Can you work these out from the model? Positions are in its coordinate system, mm. A direction names the side the tool comes from. Round coordinates to 2 decimals unless told otherwise and drop trailing zeros. Order: outer loops, then holes, each group sorted by start corner. A loop starts at its lowest first (then second) coordinate and runs counter-clockwise, first axis right, second up. Notation, with made-up numbers: M 13.25,86.5 L 36.25,86.5 A11 ccw 36.25,92.5 Z; hole C 60,42.25 d7. An arc over 180 degrees is marked long. Answer as a JSON object with one key per item and string values. Group by question number.
from build123d import *

# Parameters (mm, degrees)
SKETCH1_W           = 40
SKETCH1_H           = 50
BOSS_EXTRUDE1_DEPTH = 10
SKETCH2_W           = 40
SKETCH2_H           = 27
CUT_EXTRUDE1_DEPTH  = 1
SKETCH3_R           = 1.75
CUT_EXTRUDE2_DEPTH  = 10
SKETCH4_W           = 40
SKETCH4_H           = 20
CUT_EXTRUDE3_DEPTH  = 1
SKETCH6_R           = 2.25
CUT_EXTRUDE4_DEPTH  = 10
SKETCH7_W           = 52
SKETCH7_H           = 40
BOSS_EXTRUDE2_DEPTH = 10
SKETCH8_R           = 11
CUT_EXTRUDE5_DEPTH  = 10
SKETCH9_W           = 6
SKETCH9_H           = 10
SKETCH9_W_2         = 12
CUT_EXTRUDE6_DEPTH  = 10
SKETCH10_R          = 1.5
CUT_EXTRUDE7_DEPTH  = 10
FILLET1_R           = 1.5
FILLET2_R           = 1.5


with BuildPart() as part:
    # Sketch1 → Boss-Extrude1 (new body)
    with BuildSketch(Plane(origin=(0, 0, 0), x_dir=(0, 0, -1), z_dir=(1, 0, 0))):
        with Locations((20, 26.83908046)):
            Rectangle(SKETCH1_W, SKETCH1_H)
    extrude(amount=BOSS_EXTRUDE1_DEPTH)

    # Sketch2 → Cut-Extrude1 (cut)
    with BuildSketch(Plane.ZY):
        with Locations((-20, 15.33908046)):
            Rectangle(SKETCH2_W, SKETCH2_H)
    extrude(amount=-CUT_EXTRUDE1_DEPTH, mode=Mode.SUBTRACT)

    # Sketch3 → Cut-Extrude2 (cut)
    with BuildSketch(Plane(origin=(10, 0, 0), x_dir=(0, 0, -1), z_dir=(1, 0, 0))):
        with Locations((10, 25.33908046)):
            Circle(SKETCH3_R)
        with Locations((30, 25.33908046)):
            Circle(SKETCH3_R)
        with Locations((30, 5.33908046)):
            Circle(SKETCH3_R)
        with Locations((10, 5.33908046)):
            Circle(SKETCH3_R)
    extrude(amount=-CUT_EXTRUDE2_DEPTH, mode=Mode.SUBTRACT)

    # Sketch4 → Cut-Extrude3 (cut)
    with BuildSketch(Plane(origin=(10, 0, 0), x_dir=(0, 0, -1), z_dir=(1, 0, 0))):
        with Locations((20, 41.83908046)):
            Rectangle(SKETCH4_W, SKETCH4_H)
    extrude(amount=-CUT_EXTRUDE3_DEPTH, mode=Mode.SUBTRACT)

    # Sketch6 → Cut-Extrude4 (cut)
    with BuildSketch(Plane.ZY):
        with Locations((-30, 41.83908046)):
            Circle(SKETCH6_R)
        with Locations((-10, 41.83908046)):
            Circle(SKETCH6_R)
    extrude(amount=-CUT_EXTRUDE4_DEPTH, mode=Mode.SUBTRACT)

    # Sketch7 → Boss-Extrude2 (add)
    with BuildSketch(Plane(origin=(0, 51.83908046, 0), x_dir=(1, 0, 0), z_dir=(0, 1, 0))):
        with Locations((-16, 20)):
            Rectangle(SKETCH7_W, SKETCH7_H)
    extrude(amount=BOSS_EXTRUDE2_DEPTH)

    # Sketch8 → Cut-Extrude5 (cut)
    with BuildSketch(Plane(origin=(0, 61.83908046, 0), x_dir=(1, 0, 0), z_dir=(0, 1, 0))):
        with Locations(Location((-20.5, 20, 0), (0, 0, 270))):
            Circle(SKETCH8_R)
    extrude(amount=-CUT_EXTRUDE5_DEPTH, mode=Mode.SUBTRACT)

    # Sketch9 → Cut-Extrude6 (cut)
    with BuildSketch(Plane(origin=(9, 0, 0), x_dir=(0, 0, -1), z_dir=(1, 0, 0))):
        with Locations((37, 41.83908046)):
            Rectangle(SKETCH9_W, SKETCH9_H)
        with Locations((20, 41.83908046)):
            Rectangle(SKETCH9_W_2, SKETCH9_H)
        with Locations((3, 41.83908046)):
            Rectangle(SKETCH9_W, SKETCH9_H)
    extrude(amount=-CUT_EXTRUDE6_DEPTH, mode=Mode.SUBTRACT)

    # Sketch10 → Cut-Extrude7 (cut)
    with BuildSketch(Plane(origin=(0, 61.83908046, 0), x_dir=(1, 0, 0), z_dir=(0, 1, 0))):
        with Locations(Location((-36, 35.5, 0), (0, 0, 270))):
            Circle(SKETCH10_R)
        with Locations(Location((-5, 35.5, 0), (0, 0, 270))):
            Circle(SKETCH10_R)
        with Locations(Location((-5, 4.5, 0), (0, 0, 270))):
            Circle(SKETCH10_R)
        with Locations(Location((-36, 4.5, 0), (0, 0, 270))):
            Circle(SKETCH10_R)
    extrude(amount=-CUT_EXTRUDE7_DEPTH, mode=Mode.SUBTRACT)

    # Fillet1
    fillet1_edges = [part.edges().sort_by_distance(p)[0] for p in [
        (4.5, 36.83908046, -14),
        (4.5, 46.83908046, -14),
        (4.5, 46.83908046, -26),
        (4.5, 36.83908046, -26),
    ]]
    fillet(fillet1_edges, radius=FILLET1_R)

    # Fillet2
    fillet2_edges = [part.edges().sort_by_distance(p)[0] for p in [
        (4.5, 36.83908046, -34),
        (4.5, 46.83908046, -34),
        (4.5, 46.83908046, -6),
        (4.5, 36.83908046, -6),
    ]]
    fillet(fillet2_edges, radius=FILLET2_R)


solid = part.part
Item 1: Suppose I cut it at C-C, the plane z = -11. Write out the boundary of the cut face in (x, y).
Item 2: Suppose I cut it at B-B, the plane x = -20.5. Write out the boundary of the cut face in (y, z).
Item 3: Suppose I cut it at D-D, the plane x = -11. Write out the boundary of the cut face in (y, z), and give its area (3 significant figures).
Item 4: I'm going to push flat-ended pins straight in: pin 1 Ø5 at (y, z) = (48.5, -32) entering from +X; pin 2 Ø10 at (y, z) = (44.5, -22) entering from -X; pin 3 Ø4 at (x, z) = (-5, -4.5) entering from -Y. Where does each tip first touch, or does it pass through?
Item 5: Suppose I cut it at A-A, the plane x = -36. Write out the boundary of the cut face in (y, z), and give its area (3 significant figures).
Item 6: I need wall thicknesses on line 1 (X direction, y = 59.25, z = -35.5); line 2 (Y direction, x = 3, z = -30); line 3 (Y direction, x = 7.5, z = -3). Which ranges of each line are inside material? Lowest first, please.
Item 7: If we mould it in two halves opening along X, with no side actions, what happens to faces 1 (the face through (-5.9, 56.9, -36.7)), 2 (the face through (5, 36.839, -20)), 3 (the face through (9, 49, -20))? For each: +X half, -X half, draft (parallel to the pull), parting line (faces both ways), or undercut.
Item 8: On a 3-axis mill with a long thin cutter (end or side, diameter ignored), from which of +Z, -Z, +X, -X, +Y, -Y can I reach the whole of each face in a straight line? I mean faces 4 (the face through (5, 42, -34)), 5 (the face through (-16, 56, -40)), 6 (the face through (4.44, 37.27, -25.55)), 7 (the face through (-11, 61.839, -29)), 8 (the face through (4.44, 46.39, -5.57)). Say none if no direction works.
Computed:
{
 "1": {"outline": "M -42,51.84 L -26.82,51.84 L -26.82,61.84 L -42,61.84 Z; M -14.18,51.84 L 0,51.84 L 0,43.85 L 9,43.85 L 9,51.84 L 10,51.84 L 10,61.84 L -14.18,61.84 Z; M 0,28.84 L 1,28.84 L 1,26.78 L 10,26.78 L 10,31.84 L 9,31.84 L 9,39.82 L 0,39.82 Z; M 1,1.84 L 10,1.84 L 10,3.9 L 1,3.9 Z; M 1,6.78 L 10,6.78 L 10,23.9 L 1,23.9 Z"},
 "2": {"outline": "M 51.84,-40 L 61.84,-40 L 61.84,-31 L 51.84,-31 Z; M 51.84,-9 L 61.84,-9 L 61.84,0 L 51.84,0 Z"},
 "3": {"outline": "M 51.84,-40 L 61.84,-40 L 61.84,-25.55 L 51.84,-25.55 Z; M 51.84,-14.45 L 61.84,-14.45 L 61.84,0 L 51.84,0 Z", "area": "289 mm^2"},
 "4": {"pin 1": "stops at x = 9", "pin 2": "stops at x = 0", "pin 3": "stops at y = 51.84"},
 "5": {"outline": "M 51.84,-40 L 61.84,-40 L 61.84,-37 L 51.84,-37 Z; M 51.84,-34 L 61.84,-34 L 61.84,-6 L 51.84,-6 Z; M 51.84,-3 L 61.84,-3 L 61.84,0 L 51.84,0 Z", "area": "340 mm^2"},
 "6": {"line 1": "x = -42 to -37.5, -34.5 to -6.5, -3.5 to 10", "line 2": "y = 1.84 to 3.59, 7.09 to 23.59, 27.09 to 39.59, 44.09 to 61.84", "line 3": "y = 1.84 to 36.84, 46.84 to 61.84"},
 "7": {"face 1": "undercut", "face 2": "draft", "face 3": "+X half"},
 "8": {"face 4": "-Z, +X, -X", "face 5": "-Z, +X, -X, +Y, -Y", "face 6": "+X, -X", "face 7": "+Z, -Z, +X, -X, +Y", "face 8": "+Z, +X, -X"}
}
